from build123d import *

# Parameters (mm, degrees)
SKETCH_2_R           = 90
EXTRUDE_1_DEPTH      = 2710
EXTRUDE_2_DEPTH      = 16
SKETCH_4_R           = 11.5
CUT_EXTRUDE_1_DEPTH  = 2736.411486413
SKETCH_5_W           = 300
SKETCH_5_H           = 4
EXTRUDE_3_DEPTH      = 150
CUT_EXTRUDE_2_DEPTH  = 2736.536510449
SKETCH_7_W           = 16
SKETCH_7_H           = 260
EXTRUDE_4_DEPTH      = 255
CUT_EXTRUDE_3_DEPTH  = 2743.925445578
CUT_EXTRUDE_4_DEPTH  = 2743.925445578
SKETCH_11_R          = 11.5
CUT_EXTRUDE_5_DEPTH  = 2743.925445578
SKETCH_12_R          = 110
EXTRUDE_5_DEPTH      = 12
SKETCH_14_W          = 16
SKETCH_14_H          = 260
EXTRUDE_6_DEPTH      = 250
CUT_EXTRUDE_7_DEPTH  = 2743.925445578
CUT_EXTRUDE_8_DEPTH  = 2743.925445578
SKETCH_17_R          = 11.5
CUT_EXTRUDE_9_DEPTH  = 2743.925445578
SKETCH_18_W          = 180
SKETCH_18_H          = 16
EXTRUDE_7_DEPTH      = 167
CUT_EXTRUDE_10_DEPTH = 2748.667374338
CUT_EXTRUDE_11_DEPTH = 2748.667374338
SKETCH_21_R          = 25
CUT_EXTRUDE_12_DEPTH = 2748.667374338
SKETCH_22_W          = 180
SKETCH_22_H          = 16
EXTRUDE_8_DEPTH      = 160
SKETCH_23_W          = 244
SKETCH_23_H          = 16
EXTRUDE_9_DEPTH      = 329
CUT_EXTRUDE_13_DEPTH = 2749.286011317
CUT_EXTRUDE_14_DEPTH = 2749.286011317
SKETCH_27_R          = 20
CUT_EXTRUDE_15_DEPTH = 2749.286011317


with BuildPart() as part:
    # Sketch 2 → Extrude 1 (new body)
    with BuildSketch(Plane(origin=(0, 0, 0), x_dir=(0, 0, -1), z_dir=(1, 0, 0))):
        Circle(SKETCH_2_R)
    extrude(amount=EXTRUDE_1_DEPTH)

    # Sketch 3 → Extrude 2 (add)
    with BuildSketch(Plane(origin=(2710, 0, 0), x_dir=(0, 0, -1), z_dir=(1, 0, 0))):
        Polygon((-150, -90), (150, -90), (150, 90), (15, 170), (-15, 170), (-150, 90), align=None)
    extrude(amount=EXTRUDE_2_DEPTH)

    # Sketch 4 → Cut-Extrude 1 (cut, through all)
    with BuildSketch(Plane(origin=(2726, 0, 0), x_dir=(0, 0, -1), z_dir=(1, 0, 0))):
        with Locations((115, -40)):
            Circle(SKETCH_4_R)
        with Locations((115, 40)):
            Circle(SKETCH_4_R)
        with Locations((-115, 40)):
            Circle(SKETCH_4_R)
        with Locations((-115, -40)):
            Circle(SKETCH_4_R)
    extrude(amount=-CUT_EXTRUDE_1_DEPTH, mode=Mode.SUBTRACT)

    # Sketch 5 → Extrude 3 (add)
    with BuildSketch(Plane.ZY.offset(-2710)):
        Rectangle(SKETCH_5_W, SKETCH_5_H)
    extrude(amount=EXTRUDE_3_DEPTH)

    # Sketch 6 → Cut-Extrude 2 (cut, through all)
    with BuildSketch(Plane.XZ.offset(2)):
        Polygon((2690, 150), (2560, 109.977775034), (2560, 150), align=None)
        Polygon((2560, -109.977775034), (2560, -150), (2690, -150), align=None)
    extrude(amount=-CUT_EXTRUDE_2_DEPTH, mode=Mode.SUBTRACT)

    # Sketch 7 → Extrude 4 (add)
    with BuildSketch(Plane.ZY.offset(-2710)):
        with Locations((0, 130)):
            Rectangle(SKETCH_7_W, SKETCH_7_H)
    extrude(amount=EXTRUDE_4_DEPTH)

    # Sketch 9 → Cut-Extrude 3 (cut, through all)
    with BuildSketch(Plane(origin=(0, 0, -8), x_dir=(-1, 0, 0), z_dir=(0, 0, -1))):
        Polygon((-2710, 260), (-2500, 260), (-2710, 170), align=None)
    extrude(amount=-CUT_EXTRUDE_3_DEPTH, mode=Mode.SUBTRACT)

    # Sketch 10 → Cut-Extrude 4 (cut, through all)
    with BuildSketch(Plane(origin=(0, 0, -8), x_dir=(-1, 0, 0), z_dir=(0, 0, -1))):
        Polygon((-2500, 260), (-2455, 194), (-2455, 260), align=None)
    extrude(amount=-CUT_EXTRUDE_4_DEPTH, mode=Mode.SUBTRACT)

    # Sketch 11 → Cut-Extrude 5 (cut, through all)
    with BuildSketch(Plane(origin=(0, 0, -8), x_dir=(-1, 0, 0), z_dir=(0, 0, -1))):
        with Locations(Location((-2576.522543277, 159.619021786, 0), (0, 0, 90))):
            Circle(SKETCH_11_R)
        with Locations(Location((-2510.571491725, 204.901013782, 0), (0, 0, 90))):
            Circle(SKETCH_11_R)
    extrude(amount=-CUT_EXTRUDE_5_DEPTH, mode=Mode.SUBTRACT)

    # Sketch 12 → Extrude 5 (add)
    with BuildSketch(Plane.ZY):
        Circle(SKETCH_12_R)
    extrude(amount=EXTRUDE_5_DEPTH)

    # Sketch 14 → Extrude 6 (add)
    with BuildSketch(Plane(origin=(0, 0, 0), x_dir=(0, 0, -1), z_dir=(1, 0, 0))):
        with Locations((0, 130)):
            Rectangle(SKETCH_14_W, SKETCH_14_H)
    extrude(amount=EXTRUDE_6_DEPTH)

    # Sketch 15 → Cut-Extrude 7 (cut, through all)
    with BuildSketch(Plane(origin=(0, 0, -8), x_dir=(-1, 0, 0), z_dir=(0, 0, -1))):
        Polygon((-250, 194), (-250, 89.643739324), (-158, 89.643739324), align=None)
        Polygon((-200, 260), (0, 160), (0, 260), align=None)
    extrude(amount=-CUT_EXTRUDE_7_DEPTH, mode=Mode.SUBTRACT)

    # Sketch 16 → Cut-Extrude 8 (cut, through all)
    with BuildSketch(Plane(origin=(0, 0, -8), x_dir=(-1, 0, 0), z_dir=(0, 0, -1))):
        Polygon((-250, 260), (-200, 260), (-250, 194), align=None)
    extrude(amount=-CUT_EXTRUDE_8_DEPTH, mode=Mode.SUBTRACT)

    # Sketch 17 → Cut-Extrude 9 (cut, through all)
    with BuildSketch(Plane(origin=(0, 0, -8), x_dir=(-1, 0, 0), z_dir=(0, 0, -1))):
        with Locations(Location((-128.477456723, 159.619021786, 0), (0, 0, 90))):
            Circle(SKETCH_17_R)
        with Locations(Location((-194.428508275, 204.901013782, 0), (0, 0, 90))):
            Circle(SKETCH_17_R)
    extrude(amount=-CUT_EXTRUDE_9_DEPTH, mode=Mode.SUBTRACT)

    # Sketch 18 → Extrude 7 (add)
    with BuildSketch(Plane.ZY.offset(12)):
        with Locations((0, 42)):
            Rectangle(SKETCH_18_W, SKETCH_18_H)
        with Locations((0, -42)):
            Rectangle(SKETCH_18_W, SKETCH_18_H)
    extrude(amount=EXTRUDE_7_DEPTH)

    # Sketch 19 → Cut-Extrude 10 (cut, through all)
    with BuildSketch(Plane.XZ.offset(50)):
        with BuildLine():
            Line((-115.378912249, 74.131776965), (-12, 90))
            Line((-12, 90), (-179, 90))
            Line((-179, 90), (-179, 0))
            ThreePointArc((-179, 0), (-160.914051071, 48.844557431), (-115.378912249, 74.131776965))
        make_face()
    extrude(amount=-CUT_EXTRUDE_10_DEPTH, mode=Mode.SUBTRACT)

    # Sketch 20 → Cut-Extrude 11 (cut, through all)
    with BuildSketch(Plane.XZ.offset(50)):
        with BuildLine():
            Line((-115.378912249, -74.131776965), (-12, -90))
            Line((-12, -90), (-179, -90))
            Line((-179, -90), (-179, 0))
            ThreePointArc((-179, 0), (-160.914051071, -48.844557431), (-115.378912249, -74.131776965))
        make_face()
    extrude(amount=-CUT_EXTRUDE_11_DEPTH, mode=Mode.SUBTRACT)

    # Sketch 21 → Cut-Extrude 12 (cut, through all)
    with BuildSketch(Plane.XZ.offset(50)):
        with Locations(Location((-104, 0, 0), (0, 0, 270))):
            Circle(SKETCH_21_R)
    extrude(amount=-CUT_EXTRUDE_12_DEPTH, mode=Mode.SUBTRACT)

    # Sketch 22 → Extrude 8 (add)
    with BuildSketch(Plane.ZY.offset(12)):
        with Locations((0, 42)):
            Rectangle(SKETCH_22_W, SKETCH_22_H)
        with Locations((0, -42)):
            Rectangle(SKETCH_22_W, SKETCH_22_H)
    extrude(amount=-EXTRUDE_8_DEPTH)

    # Sketch 23 → Extrude 9 (add)
    with BuildSketch(Plane.XY.offset(105)):
        with Locations((122, 0)):
            Rectangle(SKETCH_23_W, SKETCH_23_H)
    extrude(amount=-EXTRUDE_9_DEPTH)

    # Sketch 25 → Cut-Extrude 13 (cut, through all)
    with BuildSketch(Plane(origin=(0, -8, 0), x_dir=(-1, 0, 0), z_dir=(0, -1, 0))):
        with BuildLine():
            Line((-244, 164), (-244, 224))
            Line((-244, 224), (-184, 224))
            ThreePointArc((-184, 224), (-226.426406871, 206.426406871), (-244, 164))
        make_face()
    extrude(amount=-CUT_EXTRUDE_13_DEPTH, mode=Mode.SUBTRACT)

    # Sketch 26 → Cut-Extrude 14 (cut, through all)
    with BuildSketch(Plane.XZ.offset(8)):
        with BuildLine():
            Line((148.844142163, -212.62165834), (0, -105))
            Line((0, -105), (0, -224))
            Line((0, -224), (184, -224))
            ThreePointArc((184, -224), (165.524333576, -221.084584173), (148.844142163, -212.62165834))
        make_face()
    extrude(amount=-CUT_EXTRUDE_14_DEPTH, mode=Mode.SUBTRACT)

    # Sketch 27 → Cut-Extrude 15 (cut, through all)
    with BuildSketch(Plane.XZ.offset(8)):
        with Locations((184, -164)):
            Circle(SKETCH_27_R)
    extrude(amount=-CUT_EXTRUDE_15_DEPTH, mode=Mode.SUBTRACT)


solid = part.part
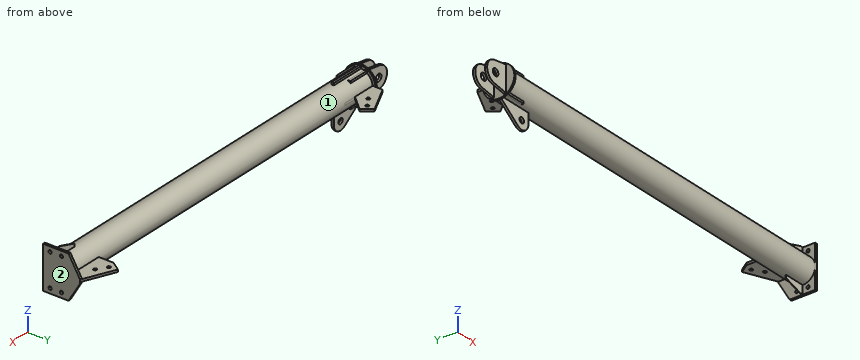
Can you work these out from the model? Positions are in its coordinate system, mm. Face numbers are marked on the shaded views. A direction names the side the tool comes from. Round coordinates to 2 decimals unless told otherwise and drop trailing zeros. Loops run counter-clockwise (first coordinate to the right, second up) from the corner with the lowest first, then second, coordinate; pieces in that order, holes last. Notation, with made-up numbers: (53.25, 55) - (108.25, 55) arc R24 cw to (108.25, 66) - close; hole circle Ø9 at (-18.75, -7). An arc over 180 degrees is marked (long way). Answer in a Markdown table with one row per item. Add a question column.
Q1. I want a section at A-A on x = 1170. List the corners of the cut face in (y, z) for me, and give its area (3 significant figures).
Q2. I need wall thicknesses on L1, parallel to X at y = -43.5, z = 0; L2, parallel to X at y = -87, z = 41.5; L3, parallel to X at y = 19.5, z = 84.5. Which ranges of each line are inside material? Lowest first, please.
Q3. Which directions (+Z, -Z, +X, -X, +Y, -Y) give clear straight access to the entire face, cutting with the end or side of a thin tool? Please do the marked faces 1 and 2.
Q4. For pin 1 Ø12 at (x, z) = (507.5, 67) entering from +Y; pin 2 Ø12 at (y, z) = (71, -8.5) entering from -X; pin 3 Ø3 at (x, y) = (1716.5, -22.5) entering from -Z; pin 4 Ø14 at (y, z) = (40, -115) entering from -X, each with a flat end and sliding along its axis, tell me the tip position at first contact or that it passes through.
A:
| question | item | result |
|---|---|---|
| 1 | outline | circle Ø180 at (0, 0) |
| 1 | area | 25,400 mm^2 |
| 2 | L1 | -179 to -129, -79 to 2726 |
| 2 | L2 | -12 to 0, 2710 to 2726 |
| 2 | L3 | -12 to 2726 |
| 3 | face 1 | none |
| 3 | face 2 | +Z, -Z, +X, +Y, -Y |
| 4 | pin 1 | y = 66.17 |
| 4 | pin 2 | x = -12 |
| 4 | pin 3 | z = -87.52 |
| 4 | pin 4 | through |
